Verification items for this drawing (mm, ordinates from the low corner). A direction names the side the tool comes from. Round coordinates to 2 decimals unless told otherwise and drop trailing zeros. Loops run counter-clockwise (first coordinate to the right, second up) from the corner with the lowest first, then second, coordinate; pieces in that order, holes last. Notation, with made-up numbers: (82, 57.5) - (124, 57.5) arc R4 cw to (124, 62.5) - close; hole circle Ø5 at (22, 84.5). An arc over 180 degrees is marked (long way). Put each result on its own line as item: value.
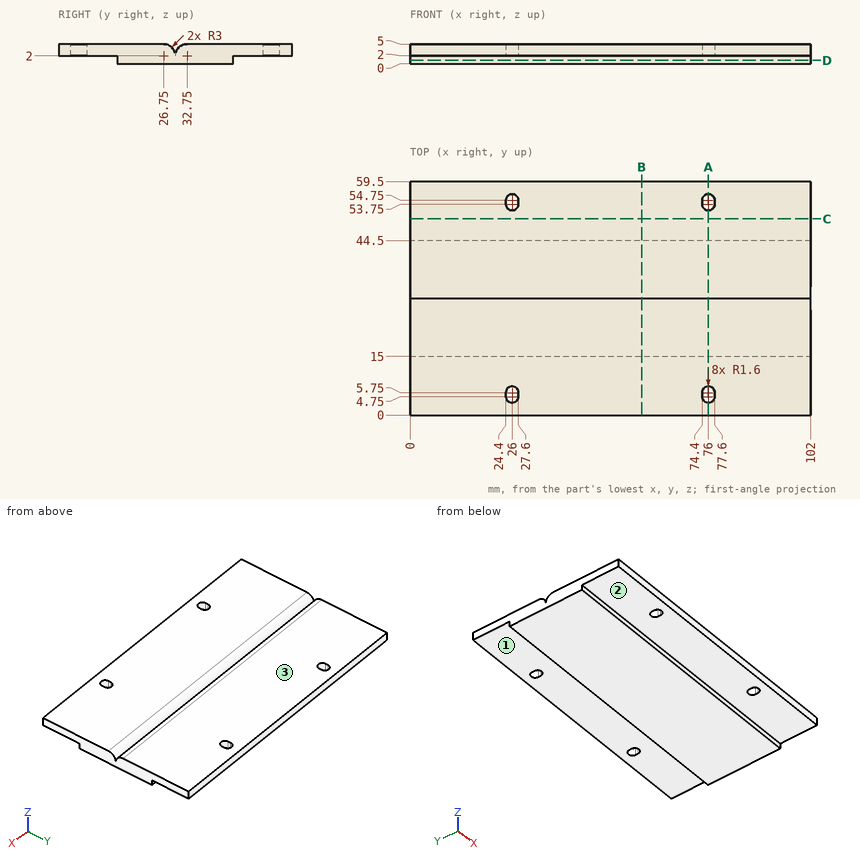
Item 1: Go/stop test with flat-tipped pins: pin 1 (0.5 mm diameter, centred on y = 54.5, z = 3, fed in from -X); pin 2 (7.5 mm diameter, centred on x = 27, y = 55.5, fed in from -Z); pin 3 (1 mm diameter, centred on x = 36, z = 1, fed in from +Y); pin 4 (0.6 mm diameter, centred on x = 75, z = 1, fed in from -Y). Record where each tip stops, or that it passes through.
Filled sheet:
pin 1: x = 0
pin 2: z = 2
pin 3: y = 44.5
pin 4: y = 15
Item 2: Section check D-D on z = 0.8. Enter the section's corners in (x, y), then the cut area to 3 significant figures.
Filled sheet:
outline: (0, 15) - (102, 15) - (102, 44.5) - (0, 44.5) - close
area: 3,010 mm²
Item 3: Section check A-A on x = 76. Enter the section's corners in (y, z).
Filled sheet:
outline: (0, 2) - (3.15, 2) - (3.15, 5) - (0, 5) - close; (7.35, 2) - (15, 2) - (15, 0) - (44.5, 0) - (44.5, 2) - (52.15, 2) - (52.15, 5) - (32.75, 5) arc R3 ccw to (29.75, 2) arc R3 ccw to (26.75, 5) - (7.35, 5) - close; (56.35, 2) - (59.5, 2) - (59.5, 5) - (56.35, 5) - close
Item 4: Thickness scan on line 1 (X direction, y = 6, z = 2.5); line 2 (X direction, y = 53, z = 4.7); line 3 (Z direction, x = 5, y = 13.5). Record the ranges inside material, lowest first. Write a range as from..to.
Filled sheet:
line 1: 0..24.42, 27.58..74.42, 77.58..102
line 2: 0..24.59, 27.41..74.59, 77.41..102
line 3: 2..5
Item 5: Tool access check on the marked faces 1, 2 and 3. Record the directions out of +Z, -Z, +X, -X, +Y, -Y that give a thin tool (end or side, any length) a straight path to the whole face; none if there is none.
Filled sheet:
face 1: -Z, +X, -X, +Y
face 2: -Z, +X, -X, -Y
face 3: +Z, +X, -X, +Y, -Y
Item 6: Section check B-B on x = 59. Enter the section's corners in (y, z), then the cut area to 3 significant figures.
Filled sheet:
outline: (0, 2) - (15, 2) - (15, 0) - (44.5, 0) - (44.5, 2) - (59.5, 2) - (59.5, 5) - (32.75, 5) arc R3 ccw to (29.75, 2) arc R3 ccw to (26.75, 5) - (0, 5) - close
area: 234 mm²
Item 7: Section check C-C on y = 50. Enter the section's corners in (x, z).
Filled sheet:
outline: (0, 2) - (102, 2) - (102, 5) - (0, 5) - close
